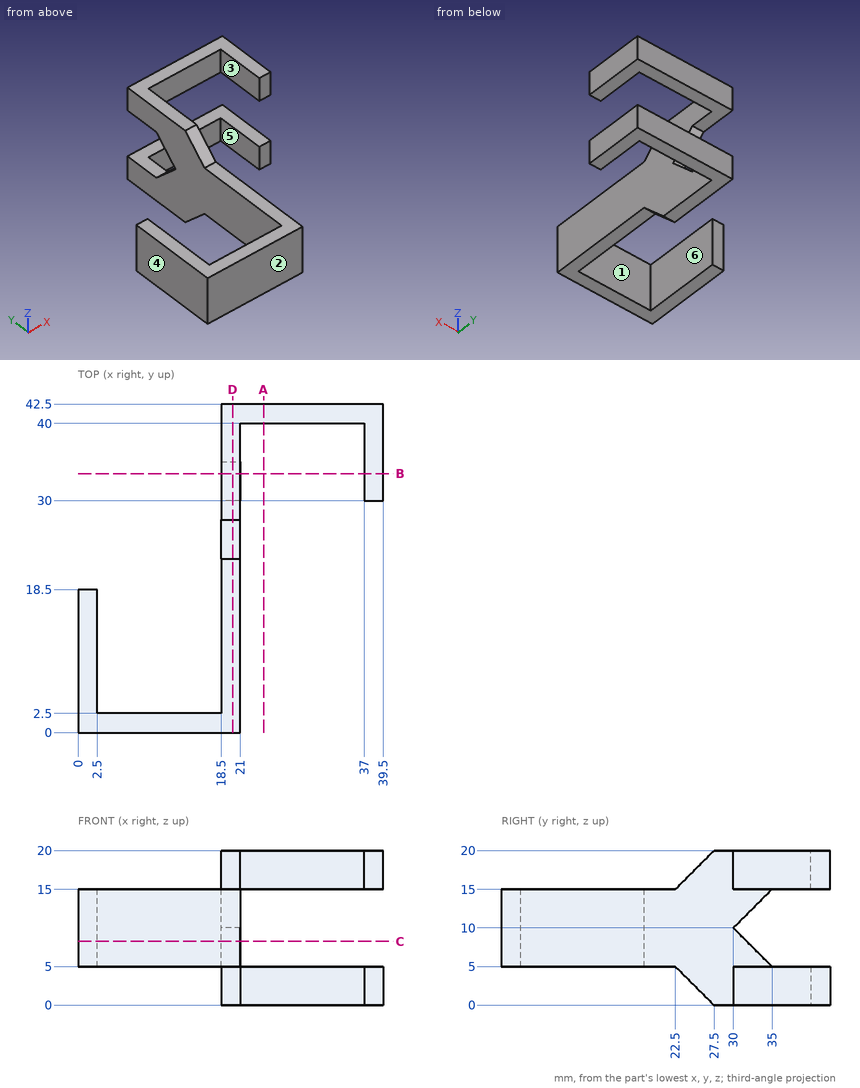
Design review of the part shown in the three views and the two pictorial views. Dimensions are in mm from the part's minimum x, y and z. A direction names the side the tool comes from. Round coordinates to 2 decimals unless told otherwise and drop trailing zeros. Loops run counter-clockwise (first coordinate to the right, second up) from the corner with the lowest first, then second, coordinate; pieces in that order, holes last. Notation, with made-up numbers: (70, 37) -> (116, 37) arc R20 cw to (116, 41) -> close; hole circle Ø4 at (14.25, -26.75). An arc over 180 degrees is marked (long way). Return JSON: item names as keys, results as strings.
(1) Add section A-A on x = 24. Write out the cut boundary in (y, z).
Solved:
{"outline": "(40, 0) -> (42.5, 0) -> (42.5, 5) -> (40, 5) -> close; (40, 15) -> (42.5, 15) -> (42.5, 20) -> (40, 20) -> close"}
(2) For pin 1 (6 mm diameter, centred on y = 29, z = 10, fed in from -X); pin 2 (11 mm diameter, centred on y = 12.5, z = 10.5, fed in from +X); pin 3 (2 mm diameter, centred on x = 0.5, z = 12.5, fed in from +Y); pin 4 (3 mm diameter, centred on y = 17.5, z = 3, fed in from -X), all flat-tipped, find the tip position at first contact; note any pin that passes through.
Solved:
{"pin 1": "x = 18.5", "pin 2": "x = 21", "pin 3": "y = 18.5", "pin 4": "through"}
(3) Add section D-D on x = 20. Write out the cut boundary in (y, z), plus the area to 3 significant figures.
Solved:
{"outline": "(0, 5) -> (22.5, 5) -> (27.5, 0) -> (42.5, 0) -> (42.5, 5) -> (35, 5) -> (30, 10) -> (35, 15) -> (42.5, 15) -> (42.5, 20) -> (27.5, 20) -> (22.5, 15) -> (0, 15) -> close", "area": "500 mm2"}
(4) The part is to be moulded in two halves that separate along Y. For the marked faces 1, 2 and 3, say which applies: released by +Y, released by -Y, zero draft, split by the parting line, or undercut.
Solved:
{"face 1": "released by +Y", "face 2": "released by -Y", "face 3": "zero draft"}
(5) For the marked faces 4, 5 and 6, list the 3-axis set-ups (+Z, -Z, +X, -X, +Y, -Y) from which the entire face can be reached by the end or side of a thin tool; tool diameter is ignored.
Solved:
{"face 4": "+Z, -Z, -X, +Y, -Y", "face 5": "+Z, -Z, -Y", "face 6": "+Z, -Z, +Y"}
(6) Add section B-B on y = 33.5. Write out the cut boundary in (x, z), plus the area to 3 significant figures.
Solved:
{"outline": "(18.5, 0) -> (21, 0) -> (21, 6.5) -> (18.5, 6.5) -> close; (18.5, 13.5) -> (21, 13.5) -> (21, 20) -> (18.5, 20) -> close; (37, 0) -> (39.5, 0) -> (39.5, 5) -> (37, 5) -> close; (37, 15) -> (39.5, 15) -> (39.5, 20) -> (37, 20) -> close", "area": "57.5 mm2"}
(7) Add section C-C on z = 8.25. Write out the cut boundary in (x, y), plus the area to 3 significant figures.
Solved:
{"outline": "(0, 0) -> (21, 0) -> (21, 31.75) -> (18.5, 31.75) -> (18.5, 2.5) -> (2.5, 2.5) -> (2.5, 18.5) -> (0, 18.5) -> close", "area": "166 mm2"}
(8) For line 1 (X direction, y = 17.5, z = 8.25); line 2 (Y direction, x = 4, z = 5.5); line 3 (X direction, y = 20, z = 6.5), list the stretches that pass through material, from the lowest coordinate up.
Solved:
{"line 1": "0 to 2.5, 18.5 to 21", "line 2": "0 to 2.5", "line 3": "18.5 to 21"}
